```python
from build123d import *

# Parameters (mm, degrees)
F0_W      = 85
F0_H      = 120
F1_DEPTH  = 8.75
F2_W      = 81
F2_H      = 118
F3_DEPTH  = 6.75
F5_DEPTH  = 25
F6_W      = 1
F6_H      = 10
F7_DEPTH  = 6.75
F8_W      = 1
F8_H      = 10
F9_DEPTH  = 6.75
F10_W     = 1
F10_H     = 10
F11_DEPTH = 6.75
F12_W     = 1
F12_H     = 10
F13_DEPTH = 6.75


with BuildPart() as f1:
    # F0 (on Top) → F1 (new body)
    with BuildSketch(Plane.XY):
        Rectangle(F0_W, F0_H)
    extrude(amount=F1_DEPTH)

    # F2 (on face) → F3 (cut)
    with BuildSketch(Plane.XY.offset(8.75)):
        with Locations((0, 1)):
            Rectangle(F2_W, F2_H)
    extrude(amount=-F3_DEPTH, mode=Mode.SUBTRACT)

    # F4 (on face) → F5 (cut)
    with BuildSketch(Plane.XY.offset(8.75)):
        with BuildLine():
            Line((-10, -10), (-10, -60))
            Line((-10, -60), (10, -60))
            Line((10, -60), (10, -10))
            ThreePointArc((10, -10), (0, 0), (-10, -10))
        make_face()
    extrude(amount=-F5_DEPTH, mode=Mode.SUBTRACT)

    # F6 (on face) → F7 (cut)
    with BuildSketch(Plane.XY.offset(8.75)):
        with Locations((-41, 40)):
            Rectangle(F6_W, F6_H)
    extrude(amount=-F7_DEPTH, mode=Mode.SUBTRACT)

    # F8 (on face) → F9 (cut)
    with BuildSketch(Plane.XY.offset(8.75)):
        with Locations((41, -40)):
            Rectangle(F8_W, F8_H)
    extrude(amount=-F9_DEPTH, mode=Mode.SUBTRACT)

    # F10 (on face) → F11 (join)
    with BuildSketch(Plane.XY.offset(8.75)):
        with Locations((-41, -40)):
            Rectangle(F10_W, F10_H)
    extrude(amount=F11_DEPTH)

    # F12 (on face) → F13 (join)
    with BuildSketch(Plane.XY.offset(8.75)):
        with Locations((41, 40)):
            Rectangle(F12_W, F12_H)
    extrude(amount=F13_DEPTH)


solid = f1.part
```
Verification items for the finished model (mm, model axes). A direction names the side the tool comes from. Give positions to 0.01 mm unless a question says otherwise; leave off trailing zeros. Order: outer loops, then holes, each group sorted by start corner. A loop starts at its lowest first (then second) coordinate and runs counter-clockwise, first axis right, second up. Notation, with made-up numbers: M 78.25,76 L 87.25,76 A22 ccw 87.25,105 Z; hole C 48.5,45.25 d5. An arc over 180 degrees is marked long. Return JSON: item names as keys, results as strings. Group by question number.
1) Access from +Z, -Z, +X, -X, +Y, -Y to the whole of each face (thin tool, end or side, straight path). Record for faces 1 (the face through (41.5, -40, 5)), 2 (the face through (40.5, 12, 6)), 3 (the face through (-10, -37, 1)).
2) Section check B-B on z = 6. Record the cut outline in (x, y), and give its area (3 significant figures).
3) Section check A-A on y = -47.5. Record the cut outline in (x, z).
4) Go/stop test with flat-tipped pins: pin 1 Ø5 at (y, z) = (-34, 12.5) entering from +X; pin 2 Ø8 at (x, y) = (12.5, 24.5) entering from -Z; pin 3 Ø1.1 at (x, z) = (-41, 13) entering from +Y; pin 4 Ø5 at (y, z) = (-44, 13) entering from -X. Record where each tip stops, or that it passes through.
5) Section check C-C on y = 48. Record the cut outline in (x, z).
6) Mould release check, pull along X, two halves, no side actions. Record for faces 4 (the face through (-42.5, -1, 4)), 5 (the face through (42, 0, 8.75)), 6 (the face through (10, -38.8, 1.8)): pulls with the +X half, pulls with the -X half, needs draft (parallel to the pull), parting line crosses it, or undercut.
7) Scan lines: line 1 (X direction, y = 50.5, z = 8.25); line 2 (X direction, y = -21, z = 1.25); line 3 (Z direction, x = -29, y = 35). Record each from-to range of solid material in increasing order.
8) Section check D-D on x = 22.5. Record the cut outline in (y, z), and give its area (4 significant figures).
Answer block:
{
 "1": {"face 1": "+Z", "face 2": "+Z, +Y", "face 3": "+Z, -Z, -Y"},
 "2": {"outline": "M -42.5,-60 L -10,-60 L -10,-58 L -40.5,-58 L -40.5,35 L -41.5,35 L -41.5,45 L -40.5,45 L -40.5,60 L -42.5,60 Z; M 10,-60 L 42.5,-60 L 42.5,60 L 40.5,60 L 40.5,-35 L 41.5,-35 L 41.5,-45 L 40.5,-45 L 40.5,-58 L 10,-58 Z", "area": "582 mm^2"},
 "3": {"outline": "M -42.5,0 L -10,0 L -10,2 L -40.5,2 L -40.5,8.75 L -42.5,8.75 Z; M 10,0 L 42.5,0 L 42.5,8.75 L 40.5,8.75 L 40.5,2 L 10,2 Z"},
 "4": {"pin 1": "stops at x = -40.5", "pin 2": "stops at z = 0", "pin 3": "stops at y = -35", "pin 4": "stops at x = -41.5"},
 "5": {"outline": "M -42.5,0 L 42.5,0 L 42.5,8.75 L 40.5,8.75 L 40.5,2 L -40.5,2 L -40.5,8.75 L -42.5,8.75 Z"},
 "6": {"face 4": "pulls with the -X half", "face 5": "needs draft", "face 6": "undercut"},
 "7": {"line 1": "x = -42.5 to -40.5, 40.5 to 42.5", "line 2": "x = -42.5 to -10, 10 to 42.5", "line 3": "z = 0 to 2"},
 "8": {"outline": "M -60,0 L 60,0 L 60,2 L -58,2 L -58,8.75 L -60,8.75 Z", "area": "253.5 mm^2"}
}
